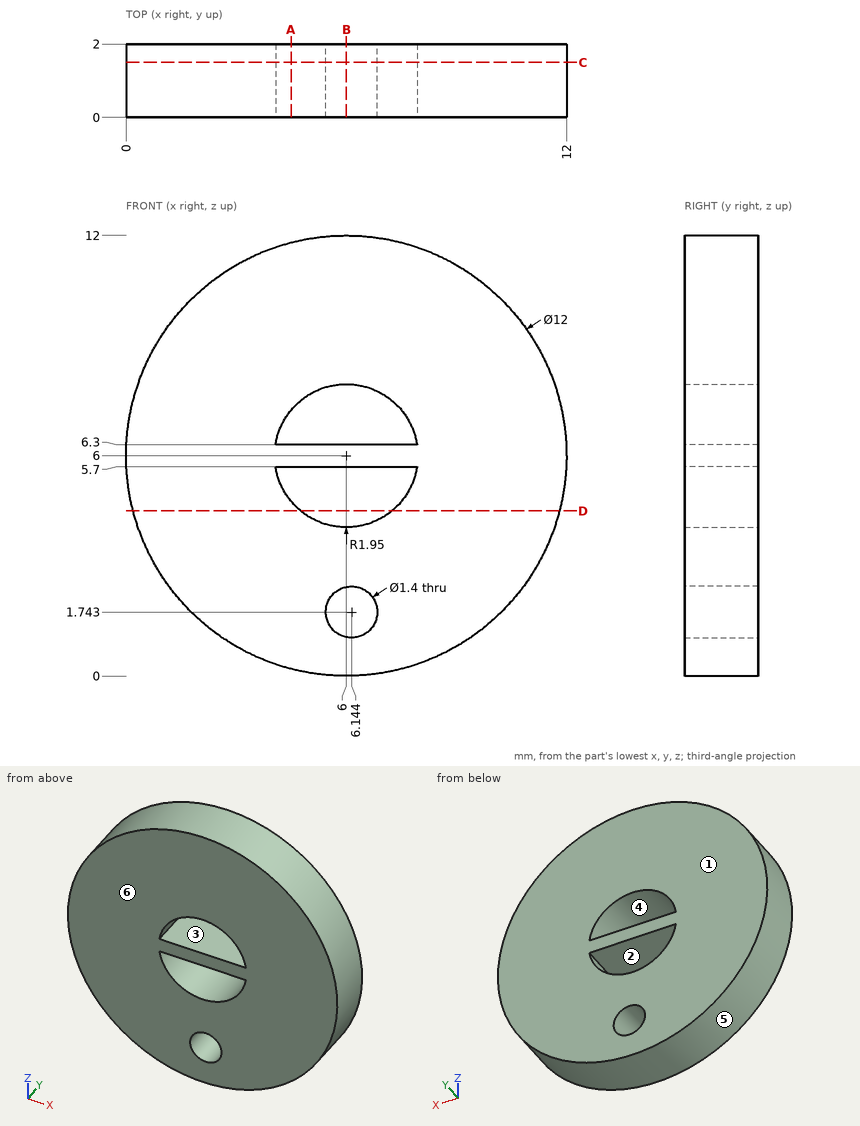
Verification items for this drawing (mm, ordinates from the low corner). A direction names the side the tool comes from. Coordinates: 2 decimals unless noted, no trailing zeros. Order: outer loops, then holes, each group sorted by start corner. A loop starts at its lowest first (then second) coordinate and runs counter-clockwise, first axis right, second up. Notation, with made-up numbers: (29.25, 34) - (44.25, 34) arc R30 cw to (44.25, 70) - close; hole circle Ø4 at (4, 5). An arc over 180 degrees is marked (long way). Use one line per item in the form item = value.
1. Section check D-D (z = 4.5). Record the boundary of the cut face in (x, y).
Here are the results:
outline = (0.19, 0) - (4.75, 0) - (4.75, 2) - (0.19, 2) - close; (7.25, 0) - (11.81, 0) - (11.81, 2) - (7.25, 2) - close
2. Access from +Z, -Z, +X, -X, +Y, -Y to the whole of each face (thin tool, end or side, straight path). Record for the marked faces 1 and 2.
Here are the results:
face_1 = +Z, -Z, +X, -X, +Y
face_2 = +Y, -Y
3. Draft check along Z on the marked faces 3, 4, 5 and 6. Enter one of: pulls with the +Z half, pulls with the -Z half, needs draft (parallel to the pull), parting line crosses it, or undercut.
Here are the results:
face_3 = undercut
face_4 = undercut
face_5 = parting line crosses it
face_6 = needs draft
4. Gauge pin test, flat ends, axial feed: pin 1 (0.6 mm diameter, centred on x = 5.5, y = 1, fed in from -Z); pin 2 (0.8 mm diameter, centred on x = 6.14, z = 1.74, fed in from -Y); pin 3 (1 mm diameter, centred on x = 6.5, y = 0.5, fed in from +Z). Record the tip position at first contact, or that the pin passes through.
Here are the results:
pin_1 = 0
pin_2 = through
pin_3 = 12
5. Section check C-C (y = 1.5). Record the boundary of the cut face in (x, z), then the cut area to 3 significant figures.
Here are the results:
outline = circle Ø12 at (6, 6); hole (4.07, 5.7) arc R1.95 ccw to (7.93, 5.7) - close; hole (4.07, 6.3) - (7.93, 6.3) arc R1.95 ccw to start; hole circle Ø1.4 at (6.14, 1.74)
area = 102 mm²
6. Scan lines: line 1 (Z direction, x = 5.75, y = 0.85) (1 decimal); line 2 (Z direction, x = 7, y = 0.9) (1 decimal); line 3 (X direction, y = 0.9, z = 7.75). Record each from-to range of solid material in increasing order.
Here are the results:
line_1 = 0 to 1.2, 2.3 to 4.1, 5.7 to 6.3, 7.9 to 12
line_2 = 0.1 to 4.3, 5.7 to 6.3, 7.7 to 11.9
line_3 = 0.26 to 5.14, 6.86 to 11.74
7. Section check B-B (x = 6). Record the boundary of the cut face in (y, z).
Here are the results:
outline = (0, 0) - (2, 0) - (2, 1.06) - (0, 1.06) - close; (0, 2.43) - (2, 2.43) - (2, 4.05) - (0, 4.05) - close; (0, 5.7) - (2, 5.7) - (2, 6.3) - (0, 6.3) - close; (0, 7.95) - (2, 7.95) - (2, 12) - (0, 12) - close
8. Section check A-A (x = 4.5). Record the boundary of the cut face in (y, z).
Here are the results:
outline = (0, 0.19) - (2, 0.19) - (2, 4.75) - (0, 4.75) - close; (0, 5.7) - (2, 5.7) - (2, 6.3) - (0, 6.3) - close; (0, 7.25) - (2, 7.25) - (2, 11.81) - (0, 11.81) - close
